Source: CAD feature listing. Evaluate the final solid. Frame: model axes, mm. Face numbers are marked on the shaded views. Coordinates: 2 decimals unless noted, no trailing zeros. Order: outer loops, then holes, each group sorted by start corner. A loop starts at its lowest first (then second) coordinate and runs counter-clockwise, first axis right, second up.
Item 1: Section C-C on y = -20. Return the cut outline in (x, z).
Item 2: Ray query, line 1 (X direction, y = -26, z = 4.5); line 2 (X direction, y = -15.25, z = 2.5); line 3 (X direction, y = -10.75, z = 7.5). Return the intervals inside material, ascending.
Item 3: Section A-A on y = -9.5. Return the cut outline in (x, z), then the cut area to 3 significant figures.
Item 4: Section B-B on z = 6.35. Return the cut outline in (x, y).
Item 5: Mould query, pull axis X, two halves, no side actions, for the marked faces 1, 2, 3 and 4. Classes: released by +X, released by -X, zero draft, split by the parting line, or undercut.
Item 6: Section D-D on z = 11. Return the cut outline in (x, y).
from build123d import *

# Parameters (mm, degrees)
BOSS_EXTRUDE1_DEPTH = 12.7
SKETCH2_R           = 2.1828125
CUT_EXTRUDE1_DEPTH  = 43.777251848


with BuildPart() as part:
    # Sketch1 → Boss-Extrude1 (new body)
    with BuildSketch(Plane.XY):
        with BuildLine():
            Line((-19.123353673, -2.54), (-31.9913, -2.54))
            Line((-31.9913, -2.54), (-31.9913, -27.94))
            Line((-31.9913, -27.94), (31.9913, -27.94))
            Line((31.9913, -27.94), (31.9913, -2.54))
            Line((31.9913, -2.54), (19.123353673, -2.54))
            ThreePointArc((19.123353673, -2.54), (0, -19.2913), (-19.123353673, -2.54))
        make_face()
    extrude(amount=BOSS_EXTRUDE1_DEPTH)

    # Sketch2 → Cut-Extrude1 (cut, through all)
    with BuildSketch(Plane.XZ.offset(27.94)):
        with Locations((-25.6413, 6.35)):
            Circle(SKETCH2_R)
        with Locations((25.6413, 6.35)):
            Circle(SKETCH2_R)
    extrude(amount=-CUT_EXTRUDE1_DEPTH, mode=Mode.SUBTRACT)


solid = part.part
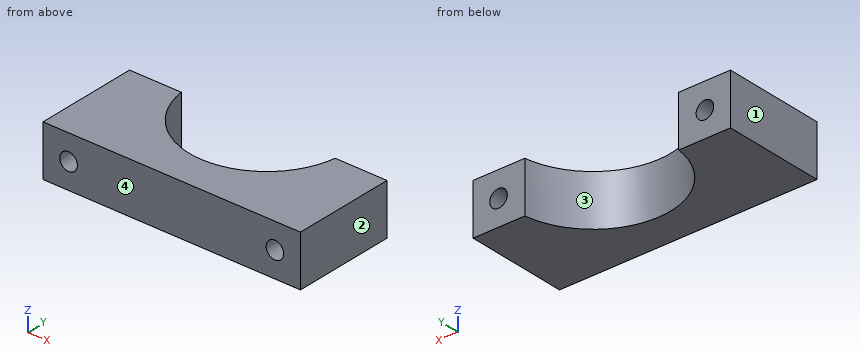
Answer list:
1. outline: (-31.99, 0) - (31.99, 0) - (31.99, 12.7) - (-31.99, 12.7) - close; hole circle Ø4.37 at (-25.64, 6.35); hole circle Ø4.37 at (25.64, 6.35)
2. line 1: x = -31.99 to -26.8, -24.48 to 24.48, 26.8 to 31.99
2. line 2: x = -31.99 to -11.81, 11.81 to 31.99
2. line 3: x = -31.99 to -27.5, -23.79 to -16.02, 16.02 to 23.79, 27.5 to 31.99
3. outline: (-31.99, 0) - (-16.79, 0) - (-16.79, 12.7) - (-31.99, 12.7) - close; (16.79, 0) - (31.99, 0) - (31.99, 12.7) - (16.79, 12.7) - close; hole circle Ø4.37 at (-25.64, 6.35); hole circle Ø4.37 at (25.64, 6.35)
3. area: 356 mm2
4. outline: (-31.99, -27.94) - (-27.82, -27.94) - (-27.82, -2.54) - (-31.99, -2.54) - close; (-23.46, -27.94) - (23.46, -27.94) - (23.46, -2.54) - (19.12, -2.54) arc R19.29 cw to (-19.12, -2.54) - (-23.46, -2.54) - close; (27.82, -27.94) - (31.99, -27.94) - (31.99, -2.54) - (27.82, -2.54) - close
5. face 1: released by -X
5. face 2: released by +X
5. face 3: undercut
5. face 4: zero draft
6. outline: (-31.99, -27.94) - (31.99, -27.94) - (31.99, -2.54) - (19.12, -2.54) arc R19.29 cw to (-19.12, -2.54) - (-31.99, -2.54) - close
